Check sheet for the modelled part. Datum: model origin and axes. Units: mm. A direction names the side the tool comes from. Give positions to 0.01 mm unless a question says otherwise; leave off trailing zeros. Write each loop counter-clockwise with the first axis right and the second up, starting at its lowest first coordinate (ties: lowest second). Pieces come first, ordered by that corner, then holes. Notation, with made-up numbers: M 24.25,-9.75 L 43.25,-9.75 A14 ccw 43.25,-3.75 Z; hole C 42.25,82.25 d11. An arc over 180 degrees is marked long. Use CSV: the item, a comma, the result in double quotes. Start each with the question number.
1. Depth check by flat-ended pin: P1, Ø1, axis at x = 1, z = -1, coming from the -Y side; P2, Ø1.6, axis at y = 10, z = 0.5, coming from the +X side. Enter the tip coordinate at first touch or a pass-through.
2. Mould release check, pull along Y, two halves, no side actions. Record for faces 1 (the face through (0, 12, 0)), 2 (the face through (-1, 0, 0)), 3 (the face through (-1, 10, 0)): +Y half, -Y half, draft (parallel to the pull), parting line (faces both ways), or undercut.
3. Cross-section at C-C, the plane y = 10. Enter the section's corners in (x, z), and give its area (4 significant figures).
4. Cross-section at A-A, the plane x = 0. Enter the section's corners in (y, z), and give its area (3 significant figures).
5. Scan lines: line 1 (Y direction, x = 0.35, z = 0); line 2 (X direction, y = 10.5, z = -0.4); line 3 (Y direction, x = 0.65, z = -1.3). Record each from-to range of solid material in increasing order.
6. Access from +Z, -Z, +X, -X, +Y, -Y to the whole of each face (thin tool, end or side, straight path). Record for faces 4 (the face through (-2, 6, 0)), 5 (the face through (1, 11, 0)), 6 (the face through (-0.7, -1.5, 0)).
7. Cross-section at B-B, the plane z = 0. Enter the section's corners in (x, y).
8. Cross-section at D-D, the plane x = -1.7. Enter the section's corners in (y, z).
from build123d import *

# Parameters (mm, degrees)
SKETCH2_W           = 4
SKETCH2_H           = 4
BOSS_EXTRUDE1_DEPTH = 12
SKETCH3_R           = 0.7
BOSS_EXTRUDE2_DEPTH = 3
SKETCH4_R           = 1
CUT_EXTRUDE1_DEPTH  = 3


with BuildPart() as part:
    # Sketch2 → Boss-Extrude1 (new body)
    with BuildSketch(Plane(origin=(0, 0, 0), x_dir=(1, 0, 0), z_dir=(0, 1, 0))):
        Rectangle(SKETCH2_W, SKETCH2_H)
    extrude(amount=BOSS_EXTRUDE1_DEPTH)

    # Sketch3 → Boss-Extrude2 (add)
    with BuildSketch(Plane(origin=(0, 0, 0), x_dir=(1, 0, 0), z_dir=(0, 1, 0))):
        Circle(SKETCH3_R)
    extrude(amount=-BOSS_EXTRUDE2_DEPTH)

    # Sketch4 → Cut-Extrude1 (cut)
    with BuildSketch(Plane(origin=(2, 0, 0), x_dir=(0, 0, -1), z_dir=(1, 0, 0))):
        with Locations((0, 10)):
            Circle(SKETCH4_R)
    extrude(amount=-CUT_EXTRUDE1_DEPTH, mode=Mode.SUBTRACT)


solid = part.part
Worked answers:
1,P1,"stops at y = 0"
1,P2,"stops at x = 2"
2,face 1,"+Y half"
2,face 2,"-Y half"
2,face 3,"undercut"
3,outline,"M -2,-2 L 2,-2 L 2,-1 L -1,-1 L -1,1 L 2,1 L 2,2 L -2,2 Z"
3,area,"10.00 mm^2"
4,outline,"M -3,-0.7 L 0,-0.7 L 0,-2 L 12,-2 L 12,2 L 0,2 L 0,0.7 L -3,0.7 Z; hole C 10,0 d2"
4,area,"49.1 mm^2"
5,line 1,"y = -3 to 9, 11 to 12"
5,line 2,"x = -2 to -1"
5,line 3,"y = 0 to 12"
6,face 4,"+Z, -Z, -X, +Y, -Y"
6,face 5,"+X"
6,face 6,"-Y"
7,outline,"M -2,0 L -0.7,0 L -0.7,-3 L 0.7,-3 L 0.7,0 L 2,0 L 2,9 L -1,9 L -1,11 L 2,11 L 2,12 L -2,12 Z"
8,outline,"M 0,-2 L 12,-2 L 12,2 L 0,2 Z"
